Autodesk Fusion 360 part; units mm, degrees
sketch "Sketch1" plane through (0, 0, 0) normal (0, 0, 1) x (1, 0, 0)
  line L0 (8.5, 17) -> (-8.5, 17)
  line L1 (-8.5, 17) -> (-8.5, -12)
  line L2 (-3.5, -17) -> (3.5, -17)
  line L3 (8.5, -12) -> (8.5, 17)
  line L4 (8.5, 17) -> (-8.5, -17) construction
  line L5 (-8.5, 17) -> (8.5, -17) construction
  line L6 (0, -17) -> (0, 17) construction
  line L7 (-3.5, 17) -> (3.5, 17)
  line L8 (8.5, 12) -> (8.5, 2)
  line L9 (8.5, 2) -> (-8.5, 2)
  line L10 (-8.5, 2) -> (-8.5, 12)
  circle A0 centre (0, -8.5) radius 4.5 construction
  line L11 (-2.0097, -4) -> (2.3533, -4) construction
  line L12 (0, 2) -> (0, 17) construction
  circle A1 centre (0, -8.5) radius 2.7
  line L13 (-8.5, 4) -> (8.5, 4)
  arc A2 (-3.5, 17) -> (-8.5, 12) centre (-3.5, 12) ccw
  arc A3 (8.5, 12) -> (3.5, 17) centre (3.5, 12) ccw
  arc A4 (3.5, -17) -> (8.5, -12) centre (3.5, -12) ccw
  arc A5 (-8.5, -12) -> (-3.5, -17) centre (-3.5, -12) ccw
  point P0 (-8.5, 17)
  point P1 (8.5, 17)
  dimension "d4" = 9
  dimension "d12" = 8.5
  dimension "d13" = 15
  dimension "d14" = 17
  dimension "d15" = 5.4
  dimension "d16" = 10.5
  dimension "d37" = 17
  dimension "d38" = 2
  dimension "d39" = 8.5
  dimension "d43" = 5
  dimension "d44" = 5
extrude "Extrude1" add sketch "Sketch1" along normal blind 2 contours L0 L1 L3 L7 L8 L10 L13 A2 A3 | L1 L3 L8 L9 L10 L13 | L1 L2 L3 L9 A4 A5
extrude "Extrude2" add sketch "Sketch1" along normal blind 6 from surface at 2 contours L1 L3 L8 L9 L10 L13
extrude "Extrude4" add sketch "Sketch1" along normal blind 2 from surface at 8 contours L0 L1 L3 L7 L8 L10 L13 A2 A3 | L1 L3 L8 L9 L10 L13
fillet "Fillet2" radius 3 2 edges at (0, 2, 10) (0, 2, 2)
fillet "Fillet2" radius 1 2 edges at (8.5, 4, 5) (-8.5, 4, 5)
equation "spacing = 4 mm"
equation "d8 = ( d4 / 2 ) + spacing"
equation "d12 = ( d4 / 2 ) + spacing"
equation "d14 = d37"
equation "d39 = d12"
equation "d44 = d43"
Verification items for the finished model (mm, model axes). A direction names the side the tool comes from. Coordinates: 2 decimals unless noted, no trailing zeros. Loops run counter-clockwise (first coordinate to the right, second up) from the corner with the lowest first, then second, coordinate; pieces in that order, holes last. Notation, with made-up numbers: (23.25, 88.5) - (78.25, 88.5) arc R19 cw to (78.25, 125.5) - close; hole circle Ø3 at (0.25, 66.25). An arc over 180 degrees is marked (long way). Put each result on its own line as item: value.
Item 1: Section check C-C (y = 8). Enter the section's corners in (x, z), then the cut area to 3 significant figures.
Conclusion:
outline: (-8.5, 0) - (8.5, 0) - (8.5, 2) - (-8.5, 2) - close; (-8.5, 8) - (8.5, 8) - (8.5, 10) - (-8.5, 10) - close
area: 68.0 mm2
Item 2: Gauge pin test, flat ends, axial feed: pin 1 Ø4 at (x, y) = (-3, 8.5) entering from -Z; pin 2 Ø0.6 at (x, z) = (2.5, 6) entering from -Y; pin 3 Ø6 at (x, y) = (-2, -5) entering from +Z; pin 4 Ø1 at (x, z) = (-0.5, 3) entering from -Y. Record the tip position at first contact, or that the pin passes through.
Conclusion:
pin 1: stops at z = 0
pin 2: stops at y = 2
pin 3: stops at z = 2
pin 4: stops at y = 0.66
Item 3: Section check D-D (z = 5.75). Enter the section's corners in (x, y), then the cut area to 3 significant figures.
Conclusion:
outline: (-8.5, 2) - (8.5, 2) - (8.5, 3) arc R1 ccw to (7.5, 4) - (-7.5, 4) arc R1 ccw to (-8.5, 3) - close
area: 33.6 mm2
Item 4: Set-up check for faces 1 (the face through (0, 4, 5)), 2 (the face through (0, 2, 6)), 3 (the face through (-8.199, 3.715, 5.042)), 4 (the face through (8.215, 3.699, 5.042)): record each of +Z, -Z, +X, -X, +Y, -Y from which the full face is reachable in a straight line by a thin tool's end or side.
Conclusion:
face 1: +X, -X, +Y
face 2: +Z, +X, -X, -Y
face 3: -X, +Y
face 4: +X, +Y
Item 5: Section check B-B (x = 0). Enter the section's corners in (y, z), then the cut area to 3 significant figures.
Conclusion:
outline: (-17, 0) - (-11.2, 0) - (-11.2, 2) - (-17, 2) - close; (-5.8, 0) - (17, 0) - (17, 2) - (4, 2) - (4, 8) - (17, 8) - (17, 10) - (5, 10) arc R3 ccw to (2, 7) - (2, 5) arc R3 cw to (-1, 2) - (-5.8, 2) - close
area: 99.2 mm2
Item 6: Draft check along X on faces 5 (the face through (7.07, -15.5, 0.99)), 6 (the face through (1.452, -10.777, 0.986)), 7 (the face through (0, 10, 2)). Enter one of: pulls with the +X half, pulls with the -X half, needs draft (parallel to the pull), parting line crosses it, or undercut.
Conclusion:
face 5: pulls with the +X half
face 6: undercut
face 7: needs draft
Item 7: Scan lines: line 1 along Z through (x, y) = (5.5, 12.5); line 2 along Y through (x, z) = (0, 1.25); line 3 along Y through (x, z) = (-1.75, 6). Record each from-to range of solid material in increasing order.
Conclusion:
line 1: z = 0 to 2, 8 to 10
line 2: y = -17 to -11.2, -5.8 to 17
line 3: y = 2 to 4
Item 8: Section check A-A (y = -8.5). Enter the section's corners in (x, z).
Conclusion:
outline: (-8.5, 0) - (-2.7, 0) - (-2.7, 2) - (-8.5, 2) - close; (2.7, 0) - (8.5, 0) - (8.5, 2) - (2.7, 2) - close
